Design review of the part built by this model. Coordinates are the model's own, in mm. A direction names the side the tool comes from. Coordinates: 2 decimals unless noted, no trailing zeros. Order: outer loops, then holes, each group sorted by start corner. A loop starts at its lowest first (then second) coordinate and runs counter-clockwise, first axis right, second up. Notation, with made-up numbers: M 64.25,88 L 76.25,88 A26 cw 76.25,102 Z; hole C 54,-13 d10. An arc over 180 degrees is marked long. Answer as a JSON object with one key per item and string values.
from build123d import *

# Parameters (mm, degrees)
SKETCH1_W           = 33.333333334
SKETCH1_H           = 3.175
SKETCH1_W_2         = 80
SKETCH1_H_2         = 20
BOSS_EXTRUDE1_DEPTH = 3.175
FILLET1_R           = 10
SKETCH2_W           = 10
SKETCH2_H           = 3.175
CUT_EXTRUDE1_DEPTH  = 3.175


with BuildPart() as part:
    # Sketch1 → Boss-Extrude1 (new body)
    with BuildSketch(Plane.XY):
        Polygon((-50, 16.666666667), (-50, 50), (-50, 80), (50, 80), (50, 50), (46.825, 50), (46.825, 16.666666667), (50, 16.666666667), (50, -16.666666667), (46.825, -16.666666667), (-46.825, -16.666666667), (-46.825, 16.666666667), align=None)
        with Locations((0, 48.4125)):
            Rectangle(SKETCH1_W, SKETCH1_H, mode=Mode.SUBTRACT)
        with Locations((0, 65)):
            Rectangle(SKETCH1_W_2, SKETCH1_H_2, mode=Mode.SUBTRACT)
    extrude(amount=BOSS_EXTRUDE1_DEPTH)

    # Fillet1
    fillet1_edges = [part.edges().sort_by_distance(p)[0] for p in [
        (-50, 80, 1.5875),
        (50, 80, 1.5875),
    ]]
    fillet(fillet1_edges, radius=FILLET1_R)

    # Sketch2 → Cut-Extrude1 (cut)
    with BuildSketch(Plane.XY.offset(3.175)):
        with Locations((25, 51.5875)):
            Rectangle(SKETCH2_W, SKETCH2_H)
        with Locations((-41.666666667, 51.5875)):
            Rectangle(SKETCH2_W, SKETCH2_H)
        with Locations((-25, 51.5875)):
            Rectangle(SKETCH2_W, SKETCH2_H)
        with Locations((41.666666667, 51.5875)):
            Rectangle(SKETCH2_W, SKETCH2_H)
    extrude(amount=-CUT_EXTRUDE1_DEPTH, mode=Mode.SUBTRACT)


solid = part.part
1) Add section D-D (z = 1.6). Count the separate pieces of the cut face and the enclosed holes in it, and give its area (3 significant figures).
Taken from the geometry:
{"separate pieces": "1", "enclosed holes": "6", "area": "7,580 mm2"}
2) Add section A-A (x = -32.5). State the section outline as (y, z) points (3 decimals), and give its area (3 significant figures).
Taken from the geometry:
{"outline": "M -16.667,0 L 55,0 L 55,3.175 L -16.667,3.175 Z; M 75,0 L 80,0 L 80,3.175 L 75,3.175 Z", "area": "243 mm2"}
3) To check wall thickness, follow L1, parallel to Y at x = 16.5, z = 0.9 (3 decimals); L2, parallel to Y at x = -37.5, z = 1.65 (3 decimals); L3, parallel to X at y = 56, z = 0.9. State the ranges of each line that lie inside material, in increasing order.
Taken from the geometry:
{"L1": "y = -16.667 to 46.825, 50 to 55, 75 to 80", "L2": "y = -16.667 to 50, 53.175 to 55, 75 to 80", "L3": "x = -50 to -40, 40 to 50"}
4) Add section B-B (y = 48). State the section outline as (x, z) points (3 decimals).
Taken from the geometry:
{"outline": "M -50,0 L -16.667,0 L -16.667,3.175 L -50,3.175 Z; M 16.667,0 L 46.825,0 L 46.825,3.175 L 16.667,3.175 Z"}
5) Insertion check: pin 1 Ø1.6 at (x, z) = (-48, 2) entering from -Y. The pin has a flat end and moves straight along its axis. Give the tip position at first contact, or say it passes through.
Taken from the geometry:
{"pin 1": "stops at y = 16.67"}
6) Mouldability with a two-part tool opening along Y and no side actions: class faces 4 (the flat face through (1, 32, 0)), 5 (the cylindrical face through (-47.15, 76.99, 1.61)), 6 (the flat face through (-46.667, 52, 2)) as released by +Y, released by -Y, zero draft, split by the parting line, or undercut.
Taken from the geometry:
{"face 4": "zero draft", "face 5": "released by +Y", "face 6": "undercut"}
7) Add section C-C (x = 38.5). State the section outline as (y, z) points (3 decimals).
Taken from the geometry:
{"outline": "M -16.667,0 L 50,0 L 50,3.175 L -16.667,3.175 Z; M 53.175,0 L 55,0 L 55,3.175 L 53.175,3.175 Z; M 75,0 L 80,0 L 80,3.175 L 75,3.175 Z"}
8) Tool access review of faces 1 (the flat face through (-20, 52, 2)), 2 (the flat face through (-46.825, 0, 2)), 3 (the flat face through (48, 16.667, 2)): name each direction out of +Z, -Z, +X, -X, +Y, -Y from which nothing blocks a thin tool from reaching the whole face with its end or side.
Taken from the geometry:
{"face 1": "+Z, -Z", "face 2": "+Z, -Z, -X, -Y", "face 3": "+Z, -Z, +X"}
